Source: CAD feature listing. Evaluate the final solid. Frame: model axes, mm. A direction names the side the tool comes from. Coordinates: 2 decimals unless noted, no trailing zeros. Loops run counter-clockwise (first coordinate to the right, second up) from the corner with the lowest first, then second, coordinate; pieces in that order, holes last. Notation, with made-up numbers: (88, -23) - (143, -23) arc R13 ccw to (143, 0) - close; hole circle Ø6 at (58, 66). An arc over 180 degrees is marked (long way). Use CSV: the item, a comma, the result in double quotes. Start each with the question number.
```python
from build123d import *
from OCP.BRepFilletAPI import BRepFilletAPI_MakeChamfer

# Parameters (mm, degrees)
SKETCH1_R                      = 35
BOSS_EXTRUDE1_DEPTH            = 6
SKETCH2_R                      = 13.5
SKETCH2_R_2                    = 8.5
BOSS_EXTRUDE2_DEPTH            = 30
BOSS_EXTRUDE3_DEPTH            = 30
CHAMFER1_SIZE2                 = 30
CHAMFER1_SIZE                  = 15.5
CIRPATTERN2_COUNT              = 4
CHAMFER1_OF_CIRPATTERN2_SIZE   = 15.5
CHAMFER1_OF_CIRPATTERN2_SIZE_2 = 30
CUT_EXTRUDE1_START             = -30
SKETCH4_R                      = 8.5
CUT_EXTRUDE1_DEPTH             = 30
CHAMFER2_SIZE                  = 1
SKETCH5_R                      = 2.5
CUT_EXTRUDE2_DEPTH             = 30
CIRPATTERN3_COUNT              = 4


with BuildPart() as part:
    # Sketch1 → Boss-Extrude1 (new body)
    with BuildSketch(Plane.XY):
        with Locations((-80.451307138, 19.943811433)):
            Circle(SKETCH1_R)
    extrude(amount=BOSS_EXTRUDE1_DEPTH)

    # Sketch2 → Boss-Extrude2 (add)
    with BuildSketch(Plane.XY.offset(6)):
        with Locations((-80.451307138, 19.943811433)):
            Circle(SKETCH2_R)
        with Locations((-80.451307138, 19.943811433)):
            Circle(SKETCH2_R_2, mode=Mode.SUBTRACT)
    extrude(amount=BOSS_EXTRUDE2_DEPTH)

    # Sketch3 → Boss-Extrude3 (add)
    with BuildSketch(Plane.XY.offset(6)):
        Polygon((-75.035425389, 9.612362561), (-71.207426337, 12.828948213), (-56.664525181, -4.478289297), (-60.492524233, -7.694874949), align=None)
    boss_extrude3 = extrude(amount=BOSS_EXTRUDE3_DEPTH)

    # Chamfer1
    chamfer1_edges = [part.edges().sort_by_distance(p)[0] for p in [
        (-58.578524707, -6.086582123, 36),
    ]]
    chamfer1_side = [part.faces().sort_by_distance(p)[0] for p in [
        (-58.777953017, -5.849246182, 36),
    ]]
    chamfer(chamfer1_edges, length=CHAMFER1_SIZE - 0.0001, length2=CHAMFER1_SIZE2 - 0.0001, reference=chamfer1_side[0])  # a hair under: the kernel refuses the full size

    # CirPattern2: Boss-Extrude3 ×4 about axis
    cirpattern2_axis = Axis((-80.451307138, 19.943811433, 0), (0, 0, 1))
    for i in range(1, CIRPATTERN2_COUNT):
        add(boss_extrude3.rotate(cirpattern2_axis, i * 360 / CIRPATTERN2_COUNT))

    # Chamfer1 of CirPattern2
    chamfer1_of_cirpattern2_edges_1 = [part.edges().sort_by_distance(p)[0] for p in [
        (-54.420913581, 41.816593865, 36),
    ]]
    chamfer1_of_cirpattern2_side_1 = [part.faces().sort_by_distance(p)[0] for p in [
        (-54.658249523, 41.617165554, 36),
    ]]
    chamfer1_of_cirpattern2_edges_2 = [part.edges().sort_by_distance(p)[0] for p in [
        (-102.324089569, 45.97420499, 36),
    ]]
    chamfer1_of_cirpattern2_side_2 = [part.faces().sort_by_distance(p)[0] for p in [
        (-102.124661259, 45.736869049, 36),
    ]]
    chamfer1_of_cirpattern2_edges_3 = [part.edges().sort_by_distance(p)[0] for p in [
        (-106.481700695, -1.928970998, 36),
    ]]
    chamfer1_of_cirpattern2_side_3 = [part.faces().sort_by_distance(p)[0] for p in [
        (-106.244364753, -1.729542687, 36),
    ]]
    chamfer1_of_cirpattern2 = BRepFilletAPI_MakeChamfer(part.part.solid().wrapped)
    for e in chamfer1_of_cirpattern2_edges_1:
        chamfer1_of_cirpattern2.Add(CHAMFER1_OF_CIRPATTERN2_SIZE - 0.0001, CHAMFER1_OF_CIRPATTERN2_SIZE_2 - 0.0001, e.wrapped, chamfer1_of_cirpattern2_side_1[0].wrapped)
    for e in chamfer1_of_cirpattern2_edges_2:
        chamfer1_of_cirpattern2.Add(CHAMFER1_OF_CIRPATTERN2_SIZE - 0.0001, CHAMFER1_OF_CIRPATTERN2_SIZE_2 - 0.0001, e.wrapped, chamfer1_of_cirpattern2_side_2[0].wrapped)
    for e in chamfer1_of_cirpattern2_edges_3:
        chamfer1_of_cirpattern2.Add(CHAMFER1_OF_CIRPATTERN2_SIZE - 0.0001, CHAMFER1_OF_CIRPATTERN2_SIZE_2 - 0.0001, e.wrapped, chamfer1_of_cirpattern2_side_3[0].wrapped)
    add(Compound.cast(chamfer1_of_cirpattern2.Shape()), mode=Mode.REPLACE)  # a hair under: the kernel refuses the full size

    # Sketch4 → Cut-Extrude1 (cut)
    with BuildSketch(Plane.XY.offset(6).offset(CUT_EXTRUDE1_START)):
        with Locations((-80.451307138, 19.943811433)):
            Circle(SKETCH4_R)
    extrude(amount=CUT_EXTRUDE1_DEPTH, mode=Mode.SUBTRACT)

    # Chamfer2
    chamfer2_edges = [part.edges().sort_by_distance(p)[0] for p in [
        (-88.951307138, 19.943811433, 36),
    ]]
    chamfer(chamfer2_edges, length=CHAMFER2_SIZE)

    # Sketch5 → Cut-Extrude2 (cut)
    with BuildSketch(Plane.XY.offset(6)):
        with Locations((-106.852057297, 22.235184611)):
            Circle(SKETCH5_R)
    cut_extrude2 = extrude(amount=-CUT_EXTRUDE2_DEPTH, mode=Mode.SUBTRACT)

    # CirPattern3: Cut-Extrude2 ×4 about axis
    cirpattern3_axis = Axis((-80.451307138, 19.943811433, 0), (0, 0, 1))
    for i in range(1, CIRPATTERN3_COUNT):
        add(cut_extrude2.rotate(cirpattern3_axis, i * 360 / CIRPATTERN3_COUNT), mode=Mode.SUBTRACT)


solid = part.part
```
(1) Reachability of faces 1 (the cylindrical face through (-79.171, 33.383, 20.79)), 2 (the flat face through (-62.402, 31.845, 17.457)), 3 (the flat face through (-95.062, 4.402, 17.457)), 4 (the cylindrical face through (-93.89, 21.22, 20.79)) from +Z, -Z, +X, -X, +Y, -Y: full face, straight path, thin tool, end or side. Return the list, or none.
(2) Section A-A on z = 24. Output: boundary loops of the cut face in (x, y), plus the area to 3 significant figures.
(3) Pin query (flat end, axial travel): pin 1 Ø6 at (x, y) = (-54.05, 17.65) entering from +Z; pin 2 Ø1 at (y, z) = (41, 5) entering from +X; pin 3 Ø4 at (x, y) = (-106.85, 22.24) entering from +Z; pin 4 Ø10 at (y, z) = (33, 4) entering from +X. Return the tip coordinate at first contact, or that it passes through.
(4) Section C-C on z = 17. Output: boundary loops of the cut face in (x, y).
(5) Ray query, line 1 (Z direction, x = -54, y = 6); line 2 (X direction, y = 15, z = 31); line 3 (Y direction, x = -74.5, z = 25). Return the intervals inside material, ascending. Write a range as [from, to].
(6) Draft query along Y for faces 5 (the cylindrical face through (-81.7, 6.5, 20.8)), 6 (the flat face through (-95.99, 34.55, 17.46)), 7 (the flat face through (-65.841, 35.486, 17.457)). Return one class per face: released by +Y, released by -Y, zero draft, split by the parting line, or undercut.
(7) Section B-B on y = 2.5. Output: boundary loops of the cut face in (x, z), plus the area to 3 significant figures.
Solution:
1,face 1,"+Z, +Y"
1,face 2,"+Z, +X"
1,face 3,"+Z, -Y"
1,face 4,"+Z, -X"
2,outline,"(-100.97, 5.97) - (-97.75, 2.14) - (-89, 9.5) arc R13.5 ccw to (-73.83, 8.18) - (-66.48, -0.57) - (-62.65, 2.64) - (-70, 11.4) arc R13.5 ccw to (-68.69, 26.56) - (-59.93, 33.92) - (-63.15, 37.75) - (-71.9, 30.39) arc R13.5 ccw to (-87.07, 31.71) - (-94.43, 40.46) - (-98.26, 37.25) - (-90.9, 28.49) arc R13.5 ccw to (-92.22, 13.32) - close; hole circle Ø17 at (-80.45, 19.94)"
2,area,"571 mm²"
3,pin 1,"stops at z = 6"
3,pin 2,"stops at x = -52.12"
3,pin 3,"passes through"
3,pin 4,"stops at x = -46.39"
4,outline,"(-103.74, 3.64) - (-100.52, -0.19) - (-89, 9.5) arc R13.5 ccw to (-73.83, 8.18) - (-64.15, -3.34) - (-60.32, -0.13) - (-70, 11.4) arc R13.5 ccw to (-68.69, 26.56) - (-57.16, 36.25) - (-60.38, 40.07) - (-71.9, 30.39) arc R13.5 ccw to (-87.07, 31.71) - (-96.75, 43.23) - (-100.58, 40.01) - (-90.9, 28.49) arc R13.5 ccw to (-92.22, 13.32) - close; hole circle Ø17 at (-80.45, 19.94)"
5,line 1,"z = [0, 6]"
5,line 2,"x = [-93.01, -87.37], [-73.54, -67.89]"
5,line 3,"y = [7.83, 13.87], [26.01, 32.06]"
6,face 5,"released by -Y"
6,face 6,"undercut"
6,face 7,"released by +Y"
7,outline,"(-110.79, 0) - (-50.11, 0) - (-50.11, 6) - (-62.53, 6) - (-62.53, 23.64) - (-69.06, 31.77) - (-69.06, 6) - (-97.32, 6) - (-97.32, 25.08) - (-105.1, 13.57) - (-105.1, 6) - (-110.79, 6) - close"
7,area,"609 mm²"
